Read the model definition and answer for the solid it produces. Units are mm, in the model's axes. A direction names the side the tool comes from. Give positions to 0.01 mm unless a question says otherwise; leave off trailing zeros. Order: outer loops, then holes, each group sorted by start corner. A loop starts at its lowest first (then second) coordinate and runs counter-clockwise, first axis right, second up.
```python
from build123d import *

# Parameters (mm, degrees)
F0_R     = 35
F2_DEPTH = 7
F3_DEPTH = 7.001
F4_R     = 8
F5_DEPTH = 7
F6_R     = 3.5
F7_DEPTH = 12
F8_R     = 6
F9_DEPTH = 12.001


with BuildPart() as f2:
    # F0 (on Top) → F2 (new body)
    with BuildSketch(Plane.XY):
        Circle(F0_R)
    extrude(amount=F2_DEPTH)

    # F1 (on face) → F3 (intersect, through all)
    with BuildSketch(Plane.XY):
        with BuildLine():
            Line((0, 28), (0, 35))
            ThreePointArc((0, 35), (-24.748737, 24.748737), (-35, 0))
            Line((-35, 0), (-28, 0))
            ThreePointArc((-28, 0), (-19.79899, 19.79899), (0, 28))
        make_face()
    extrude(amount=F3_DEPTH, mode=Mode.INTERSECT)

    # F4 (on face) → F5 (join)
    with BuildSketch(Plane.XY.offset(7)):
        with Locations((0, 31.5)):
            Circle(F4_R)
    extrude(amount=-F5_DEPTH)

    # F6 (on face) → F7 (join)
    with BuildSketch(Plane.XY.offset(7)):
        with Locations((-31.5, 0)):
            Circle(F6_R)
    extrude(amount=-F7_DEPTH)

    # F8 (on face) → F9 (cut, through all)
    with BuildSketch(Plane.XY.offset(7)):
        with Locations((0, 31.5)):
            Circle(F8_R)
    extrude(amount=-F9_DEPTH, mode=Mode.SUBTRACT)


solid = f2.part
```
1) The part is cut by section C-C on y = 31.5. Determine the outline of the cut face in (x, z), and give its area (3 significant figures).
Final values:
outline: (-15.26, 0) - (-6, 0) - (-6, 7) - (-15.26, 7) - close; (6, 0) - (8, 0) - (8, 7) - (6, 7) - close
area: 78.8 mm2
2) Given pin 1 (2 mm diameter, centred on x = -26.5, z = 5.5, fed in from +Y); pin 2 (2 mm diameter, centred on y = 33, z = 4.5, fed in from +X); pin 3 (12 mm diameter, centred on x = -21.5, y = 11.5, fed in from -Z); pin 4 (7 mm diameter, centred on x = 0, y = 31.5, fed in from -Z), each flat-ended and moving along its own axis, determine where each tip first touches the part or whether it passes through.
Final values:
pin 1: stops at y = 23.97
pin 2: stops at x = 7.98
pin 3: stops at z = 0
pin 4: passes through
3) The part is cut by section B-B on z = 2.5. Determine the outline of the cut face in (x, y), and give its area (3 significant figures).
Final values:
outline: (-35, 0) arc R3.5 ccw to (-28, 0) arc R28 cw to (-6.73, 27.18) arc R8 ccw (long way) to (-7.54, 34.18) arc R35 ccw to start; hole circle Ø12 at (0, 31.5)
area: 399 mm2
4) For a pull along X with two mould halves and no side action, classify faces 1 (the face through (-22.21, 17.05, 3.45)), 2 (the face through (-27.075, 22.18, 3.451)), 3 (the face through (-18, 23, 0)) as released by +X, released by -X, zero draft, split by the parting line, or undercut.
Final values:
face 1: undercut
face 2: released by -X
face 3: zero draft
5) The part is cut by section D-D on x = -31.5. Determine the outline of the cut face in (y, z), and give its area (3 significant figures).
Final values:
outline: (-3.5, -5) - (3.5, -5) - (3.5, 0) - (15.26, 0) - (15.26, 7) - (-3.5, 7) - close
area: 166 mm2
6) A tool of negligible diameter and unlimited length cuts with its end or side. For faces 4 (the face through (-29.885, -3.105, -0.249)), 5 (the face through (-32, 0, -5)), from which of +Z, -Z, +X, -X, +Y, -Y can it reach the whole face along a straight path? Write none if from no direction.
Final values:
face 4: -Z
face 5: -Z, +X, -X, +Y, -Y
7) The part is cut by section A-A on x = 0. Determine the outline of the cut face in (y, z).
Final values:
outline: (23.5, 0) - (25.5, 0) - (25.5, 7) - (23.5, 7) - close; (37.5, 0) - (39.5, 0) - (39.5, 7) - (37.5, 7) - close
8) Consider L1, parallel to Y at x = 0, z = 5.5; L2, parallel to Z at x = -28.5, y = 17.5; L3, parallel to X at y = 29, z = 1.5. Determine where each line is inside the solid, lowest interval first.
Final values:
L1: y = 23.5 to 25.5, 37.5 to 39.5
L2: z = 0 to 7
L3: x = -19.6 to -5.45, 5.45 to 7.6
